Here's how the part is built. I have some questions about the finished solid (model axes, mm). A direction names the side the tool comes from. Give positions to 0.01 mm unless a question says otherwise; leave off trailing zeros. Order: outer loops, then holes, each group sorted by start corner. A loop starts at its lowest first (then second) coordinate and runs counter-clockwise, first axis right, second up. Notation, with made-up numbers: M 7.5,68.5 L 44.5,68.5 A20 cw 44.5,100.5 Z; hole C 41.5,62.25 d4. An arc over 180 degrees is marked long. Use one line per item in the form item = value.
from build123d import *

# Parameters (mm, degrees)
SKETCH2_R           = 60
BOSS_EXTRUDE1_DEPTH = 22.5
SKETCH3_OUTSIDE_W   = 157.114
SKETCH3_OUTSIDE_H   = 157.114
SKETCH3_OUTSIDE_W_2 = 15
SKETCH3_OUTSIDE_H_2 = 130
CUT_EXTRUDE1_DEPTH  = 15
SKETCH4_OUTSIDE_W   = 157.114
SKETCH4_OUTSIDE_H   = 157.114
SKETCH4_OUTSIDE_W_2 = 130
SKETCH4_OUTSIDE_H_2 = 15
CUT_EXTRUDE2_DEPTH  = 15
FILLET1_R           = 1.5


with BuildPart() as part:
    # Sketch2 → Boss-Extrude1 (new, symmetric)
    with BuildSketch(Plane(origin=(0, 0, 0), x_dir=(-1, 0, 0), z_dir=(0, 1, 0))):
        with Locations(Location((0, 0, 0), (0, 0, 270))):
            Circle(SKETCH2_R)
    extrude(amount=BOSS_EXTRUDE1_DEPTH, both=True)

    # Sketch3 outside → Cut-Extrude1 (cut)
    with BuildSketch(Plane(origin=(0, 22.5, 0), x_dir=(-1, 0, 0), z_dir=(0, 1, 0))):
        Rectangle(SKETCH3_OUTSIDE_W, SKETCH3_OUTSIDE_H)
        Rectangle(SKETCH3_OUTSIDE_W_2, SKETCH3_OUTSIDE_H_2, mode=Mode.SUBTRACT)
    extrude(amount=-CUT_EXTRUDE1_DEPTH, mode=Mode.SUBTRACT)

    # Sketch4 outside → Cut-Extrude2 (cut)
    with BuildSketch(Plane.XZ.offset(22.5)):
        Rectangle(SKETCH4_OUTSIDE_W, SKETCH4_OUTSIDE_H)
        Rectangle(SKETCH4_OUTSIDE_W_2, SKETCH4_OUTSIDE_H_2, mode=Mode.SUBTRACT)
    extrude(amount=-CUT_EXTRUDE2_DEPTH, mode=Mode.SUBTRACT)

    # Fillet1
    fillet1_edges = [part.edges().sort_by_distance(p)[0] for p in [
        (7.5, 7.5, 0),
        (-7.5, 7.5, 0),
        (-7.5, 15, -59.529404499),
        (7.5, 15, 59.529404499),
        (-7.5, 15, 59.529404499),
        (7.5, 15, -59.529404499),
        (60, -22.5, 0),
        (-60, -22.5, 0),
        (0, -22.5, 7.5),
        (0, -22.5, -7.5),
        (0, -7.5, 60),
        (-39.686269666, -7.5, -45),
        (0, -7.5, 7.5),
        (0, -7.5, -7.5),
        (59.529404499, -15, -7.5),
        (-59.529404499, -15, 7.5),
        (-59.529404499, -15, -7.5),
        (59.529404499, -15, 7.5),
        (-3.757374753, 22.5, -59.882235554),
        (0, 22.5, 60),
        (7.5, 22.5, 0),
        (-7.5, 22.5, 0),
        (60, 7.5, 0),
        (-60, 7.5, 0),
    ]]
    fillet(fillet1_edges, radius=FILLET1_R)


solid = part.part
Q1. I want a section at B-B on x = 0. Write out the boundary of the cut face in (y, z).
Found:
outline = M -22.5,-6 A1.5 ccw -21,-7.5 L -9,-7.5 A1.5 cw -7.5,-9 L -7.5,-58.5 A1.5 ccw -6,-60 L 21,-60 A1.5 ccw 22.5,-58.5 L 22.5,58.5 A1.5 ccw 21,60 L -6,60 A1.5 ccw -7.5,58.5 L -7.5,9 A1.5 cw -9,7.5 L -21,7.5 A1.5 ccw -22.5,6 Z
Q2. On a 3-axis mill with a long thin cutter (end or side, diameter ignored), from which of +Z, -Z, +X, -X, +Y, -Y can I reach the whole of each face in a straight line? I mean faces 1 (the face through (-1, -15, 7.5)), 2 (the face through (-1, -7.5, -28)), 3 (the face through (-28, 7.5, 1)). Say none if no direction works.
Found:
face_1 = +Z, +X, -X, -Y
face_2 = -Z, +X, -X, -Y
face_3 = +Z, -Z, -X, +Y
Q3. I'm going to push flat-ended pins straight in: pin 1 Ø12 at (x, z) = (43.5, -15) entering from -Y; pin 2 Ø3.5 at (y, z) = (13, -8.5) entering from -X; pin 3 Ø4 at (x, z) = (-17, 11.5) entering from +Y; pin 4 Ø6 at (y, z) = (-11, 34.5) entering from +X. Where does each tip first touch, or does it pass through?
Found:
pin_1 = -7.5
pin_2 = -7.5
pin_3 = 7.5
pin_4 = through
Q4. I need wall thicknesses on L1, parallel to Z at x = 9, y = 3; L2, parallel to X at y = 15, z = -48.5. Which ranges of each line are inside material? Lowest first, please.
Found:
L1 = -59.32 to 59.32
L2 = -7.5 to 7.5
Q5. I want a section at C-C on z = 0. Write out the boundary of the cut face in (x, y), then the cut area to 3 significant figures.
Found:
outline = M -60,-21 A1.5 ccw -58.5,-22.5 L 58.5,-22.5 A1.5 ccw 60,-21 L 60,6 A1.5 ccw 58.5,7.5 L 9,7.5 A1.5 cw 7.5,9 L 7.5,21 A1.5 ccw 6,22.5 L -6,22.5 A1.5 ccw -7.5,21 L -7.5,9 A1.5 cw -9,7.5 L -58.5,7.5 A1.5 ccw -60,6 Z
area = 3,820 mm²
Q6. I want a section at A-A on y = 13. Write out the boundary of the cut face in (x, z), then the cut area to 3 significant figures.
Found:
outline = M -7.5,-58.19 A1.5 ccw -6.15,-59.68 A60 ccw 6.15,-59.68 A1.5 ccw 7.5,-58.19 L 7.5,58.19 A1.5 ccw 6.15,59.68 A60 ccw -6.15,59.68 A1.5 ccw -7.5,58.19 Z
area = 1,790 mm²
